CAD build for the part. Positions are in the model's coordinates, mm. A direction names the side the tool comes from. Round coordinates to 2 decimals unless told otherwise and drop trailing zeros. Order: outer loops, then holes, each group sorted by start corner. A loop starts at its lowest first (then second) coordinate and runs counter-clockwise, first axis right, second up. Notation, with made-up numbers: M -24.75,13.5 L 25.25,13.5 A26 cw 25.25,29.5 Z; hole C 10.5,-19 d3. An arc over 180 degrees is marked long. Answer as a JSON object with one key per item and string values.
```python
from build123d import *

# Parameters (mm, degrees)
SKETCH1_R           = 8.39
BOSS_EXTRUDE1_DEPTH = 3
SKETCH2_R           = 4.5
BOSS_EXTRUDE2_DEPTH = 2.5
SKETCH3_R           = 1.125
CUT_EXTRUDE1_DEPTH  = 13.238635545
FILLET1_R           = 0.25
SKETCH6_R           = 1.275
CUT_EXTRUDE2_DEPTH  = 14.078004435
SKETCH7_R           = 3.11
CUT_EXTRUDE3_DEPTH  = 2.5
BOSS_EXTRUDE4_DEPTH = 2.5
CIRPATTERN1_COUNT   = 26


with BuildPart() as part:
    # Sketch1 → Boss-Extrude1 (new body)
    with BuildSketch(Plane(origin=(0, 0, 0), x_dir=(1, 0, 0), z_dir=(0, 1, 0))):
        with Locations(Location((0, 0, 0), (0, 0, 270))):
            Circle(SKETCH1_R)
    extrude(amount=BOSS_EXTRUDE1_DEPTH)

    # Sketch2 → Boss-Extrude2 (add)
    with BuildSketch(Plane(origin=(0, 0, 0), x_dir=(1, 0, 0), z_dir=(0, 1, 0))):
        with Locations(Location((0, 0, 0), (0, 0, 270))):
            Circle(SKETCH2_R)
    extrude(amount=-BOSS_EXTRUDE2_DEPTH)

    # Sketch3 → Cut-Extrude1 (cut, through all)
    with BuildSketch(Plane(origin=(0, 0, 0), x_dir=(1, 0, 0), z_dir=(0, 1, 0))):
        with Locations(Location((0, 6.28, 0), (0, 0, 270))):
            Circle(SKETCH3_R)
        with Locations(Location((-6.28, 0, 0), (0, 0, 270))):
            Circle(SKETCH3_R)
        with Locations(Location((0, -6.28, 0), (0, 0, 90))):
            Circle(SKETCH3_R)
        with Locations(Location((6.28, 0, 0), (0, 0, 90))):
            Circle(SKETCH3_R)
    extrude(amount=CUT_EXTRUDE1_DEPTH, mode=Mode.SUBTRACT)

    # Fillet1
    fillet1_edges = [part.edges().sort_by_distance(p)[0] for p in [
        (0, 0, -8.39),
    ]]
    fillet(fillet1_edges, radius=FILLET1_R)

    # Sketch6 → Cut-Extrude2 (cut, through all)
    with BuildSketch(Plane(origin=(0, 3, 0), x_dir=(1, 0, 0), z_dir=(0, 1, 0))):
        with Locations(Location((0, 0, 0), (0, 0, 270))):
            Circle(SKETCH6_R)
    extrude(amount=-CUT_EXTRUDE2_DEPTH, mode=Mode.SUBTRACT)

    # Sketch7 → Cut-Extrude3 (cut)
    with BuildSketch(Plane.XZ.offset(2.5)):
        with Locations(Location((0, 0, 0), (0, 0, 270))):
            Circle(SKETCH7_R)
    extrude(amount=-CUT_EXTRUDE3_DEPTH, mode=Mode.SUBTRACT)

    # Sketch8 → Boss-Extrude4 (add)
    with BuildSketch(Plane.XZ.offset(2.5)):
        with BuildLine():
            Line((2.580937562, 1.000063428), (2.97197515, 0.880119756))
            ThreePointArc((2.97197515, 0.880119756), (2.88046583, 1.126882202), (2.766961985, 1.364332277))
            Line((2.766961985, 1.364332277), (2.580937562, 1.000063428))
        make_face()
    boss_extrude4 = extrude(amount=-BOSS_EXTRUDE4_DEPTH)

    # CirPattern1: Boss-Extrude4 ×26 about axis
    cirpattern1_axis = Axis((0, 0, 0), (0, 1, 0))
    for i in range(1, CIRPATTERN1_COUNT):
        add(boss_extrude4.rotate(cirpattern1_axis, i * 360 / CIRPATTERN1_COUNT))


solid = part.part
```
Item 1: 3-axis set-ups, long thin cutter, end or side, ignore diameter. For faces 5 (the flat face through (-4, 0, 4)), 6 (the cylindrical face through (0.338, 1.479, -5.207)): which of +Z, -Z, +X, -X, +Y, -Y reach the whole face in a straight line?
Worked answers:
{"face 5": "-Y", "face 6": "+Y, -Y"}
Item 2: Saw through at A-A on y = 1.55. List the corners of the cut face in (x, z) (3 decimals).
Worked answers:
{"outline": "C 0,0 d16.78; hole C -6.28,0 d2.25; hole C 0,0 d2.55; hole C 0,-6.28 d2.25; hole C 0,6.28 d2.25; hole C 6.28,0 d2.25"}
Item 3: Drop flat-ended pins along their axis: pin 1 Ø2 at (x, y) = (2.5, 2.5) entering from +Z; pin 2 Ø3 at (x, y) = (-2, 2.5) entering from +Z; pin 3 Ø1.5 at (x, y) = (2, -1.5) entering from -Z. Give the stop position or say it passes through.
Worked answers:
{"pin 1": "stops at z = 8.25", "pin 2": "stops at z = 8.38", "pin 3": "stops at z = -4.32"}
Item 4: Saw through at B-B on y = -1.6. State how many separate pieces and enclosed holes the cut face has, and give its area (3 significant figures).
Worked answers:
{"separate pieces": "27", "enclosed holes": "1", "area": "35.5 mm2"}
Item 5: Two-plate mould, pull along X, no slides. Class faces 1 (the cylindrical face through (0.383, 1.521, 1.216)), 2 (the cylindrical face through (1.352, -1.232, 4.292)), 3 (the flat face through (0, 3, 2)), 4 (the cylindrical face through (-7.278, 1.479, 0.519)): released by +X, released by -X, zero draft, split by the parting line, or undercut.
Worked answers:
{"face 1": "undercut", "face 2": "split by the parting line", "face 3": "zero draft", "face 4": "undercut"}
Item 6: Wall check: line 1 along X through (y, z) = (1.45, 0) (3 decimals); line 2 along X through (y, z) = (-1.85, 0); line 3 along Z through (x, y) = (-0.5, 1.45). Give the ranges that are in metal, low to high. Write a range as [from, to].
Worked answers:
{"line 1": "x = [-8.39, -7.405], [-5.155, -1.275], [1.275, 5.155], [7.405, 8.39]", "line 2": "x = [-4.5, -3.11], [3.11, 4.5]", "line 3": "z = [-8.38, -7.29], [-5.27, -1.17], [1.17, 5.27], [7.29, 8.38]"}
